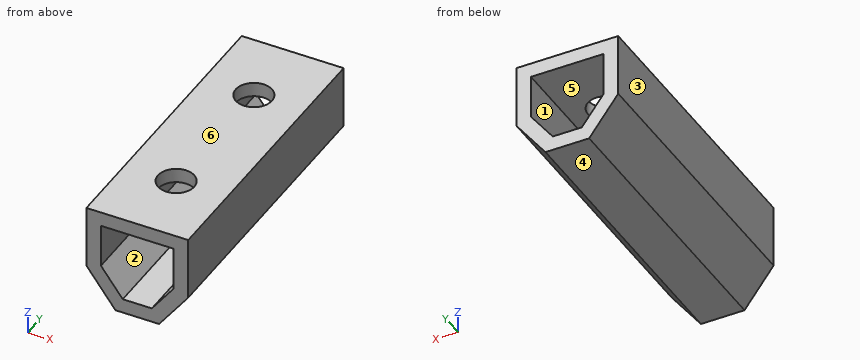
from build123d import *

# Parameters (mm, degrees)
F1_DEPTH = 10
F2_R     = 1.25
F3_DEPTH = 1


# Not quite as in the source:
# - ends of sketch curves that miss each other by under 0.0002 mm in the source are joined


with BuildPart() as f1:
    # F0 (on Front) → F1 (new body)
    with BuildSketch(Plane.XZ):
        Polygon((3.5, 6), (-3.4999988526, 6), (-3.5, 1.6666666667), (-1.5, -1), (0, -1), (1.5, -1), (3.5, 1.6666666667), align=None)
        Polygon((-2.5, 5), (0, 5), (2.5, 5), (2.5, 2), (1, 0), (0, 0), (-1, 0), (-2.5, 2), align=None, mode=Mode.SUBTRACT)
    extrude(amount=F1_DEPTH)

    # F2 (on face) → F3 (cut, through all)
    with BuildSketch(Plane.XY.offset(6)):
        with Locations((5.737e-07, -5)):
            Circle(F2_R)
    extrude(amount=-F3_DEPTH, mode=Mode.SUBTRACT)

    # F4: F1 across face


with BuildPart() as f1_1:
    add(f1.part)
    add(f1.part.mirror(Plane(origin=(4.016e-07, 0, 2.8888886977), x_dir=(1, 0, 0), z_dir=(0, 1, 0))))


solid = f1_1.part
Input: part model. Units: mm. Frame: model coordinates. Face numbers are marked on the shaded views. A direction names the side the tool comes from. Coordinates: 2 decimals unless noted, no trailing zeros. Loops run counter-clockwise (first coordinate to the right, second up) from the corner with the lowest first, then second, coordinate; pieces in that order, holes last. Notation, with made-up numbers: (-16.5, 82.5) - (18.5, 82.5) arc R11 cw to (18.5, 91.5) - close; hole circle Ø7 at (86, 83). An arc over 180 degrees is marked (long way). Answer in a Markdown table with one row per item. Add a question column.
Item 1: Section query C-C on y = -1. Return the cut outline in (x, z), then the cut area to 3 significant figures.
Item 2: Line query: line 1 along Y through (x, z) = (0, 5.4); line 2 along X through (y, z) = (6.75, 2.5); line 3 along X through (y, z) = (5, 5.6). Output: solid intervals per line, ascending. Write a range as [from, to].
Item 3: Access query for the marked faces 5 and 6. Directions: +Z, -Z, +X, -X, +Y, -Y. A direction counts if a zero-diameter tool reaches every point of the face in a straight line with its end or side. Return the directions, or none.
Item 4: Section query B-B on z = 2.75. Return the cut outline in (x, y), then the cut area to 3 significant figures.
Item 5: Mould query, pull axis X, two halves, no side actions, for the marked faces 1, 2, 3 and 4. Classes: released by +X, released by -X, zero draft, split by the parting line, or undercut.
Item 6: Section query A-A on x = 0.75. Return the cut outline in (y, z).
Item 7: Section query D-D on y = -5. Return the cut outline in (x, z).
Recorded:
| question | item | result |
|---|---|---|
| 1 | outline | (-3.5, 1.67) - (-1.5, -1) - (1.5, -1) - (3.5, 1.67) - (3.5, 6) - (-3.5, 6) - close; hole (-2.5, 2) - (-1, 0) - (1, 0) - (2.5, 2) - (2.5, 5) - (-2.5, 5) - close |
| 1 | area | 21.7 mm^2 |
| 2 | line 1 | [-10, -6.25], [-3.75, 3.75], [6.25, 10] |
| 2 | line 2 | [-3.5, -2.5], [2.5, 3.5] |
| 2 | line 3 | [-3.5, -1.25], [1.25, 3.5] |
| 3 | face 5 | +Y, -Y |
| 3 | face 6 | +Z, +X, -X, +Y, -Y |
| 4 | outline | (-3.5, -10) - (-2.5, -10) - (-2.5, 10) - (-3.5, 10) - close; (2.5, -10) - (3.5, -10) - (3.5, 10) - (2.5, 10) - close |
| 4 | area | 40.0 mm^2 |
| 5 | face 1 | undercut |
| 5 | face 2 | undercut |
| 5 | face 3 | released by -X |
| 5 | face 4 | zero draft |
| 6 | outline | (-10, -1) - (10, -1) - (10, 0) - (-10, 0) - close; (-10, 5) - (-6, 5) - (-6, 6) - (-10, 6) - close; (-4, 5) - (4, 5) - (4, 6) - (-4, 6) - close; (6, 5) - (10, 5) - (10, 6) - (6, 6) - close |
| 7 | outline | (-3.5, 1.67) - (-1.5, -1) - (1.5, -1) - (3.5, 1.67) - (3.5, 6) - (1.25, 6) - (1.25, 5) - (2.5, 5) - (2.5, 2) - (1, 0) - (-1, 0) - (-2.5, 2) - (-2.5, 5) - (-1.25, 5) - (-1.25, 6) - (-3.5, 6) - close |
